Geometry: see drawing. Coordinates: mm, zero at the bounding-box minimum. Coordinates: 2 decimals unless noted, no trailing zeros. Loops run counter-clockwise (first coordinate to the right, second up) from the corner with the lowest first, then second, coordinate; pieces in that order, holes last. Notation, with made-up numbers: (64, 82.5) -> (102, 82.5) arc R4 cw to (102, 87.5) -> close; hole circle Ø10 at (-35, -36). An arc over 180 degrees is marked (long way). Put each result on its own line as item: value. Start each with the question number.
1) Cut plane B-B (z = 3.3). Return the cut outline in (x, y), plus the area to 3 significant figures.
2) Material intervals for L1, parallel to Y at x = 45, z = 3.15; L2, parallel to X at y = 4.5, z = 3.1; L3, parallel to Y at x = 18.5, z = 2.75, sorted ascending.
3) Cut plane C-C (x = 18.5). Return the cut outline in (y, z), plus the area to 3 significant figures.
4) Cut plane A-A (x = 45). Return the cut outline in (y, z).
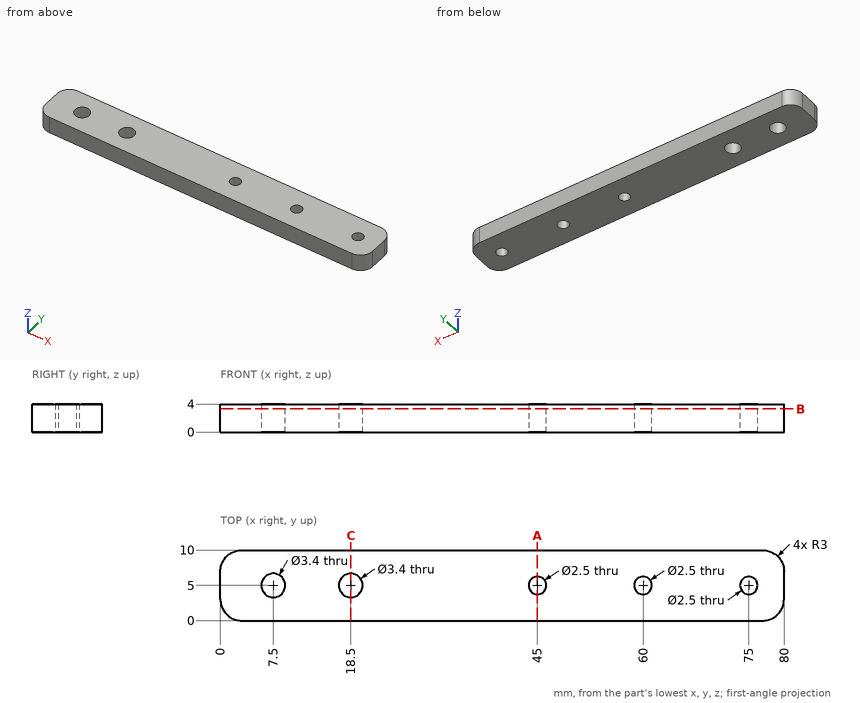
Results found:
1. outline: (0, 3) arc R3 ccw to (3, 0) -> (77, 0) arc R3 ccw to (80, 3) -> (80, 7) arc R3 ccw to (77, 10) -> (3, 10) arc R3 ccw to (0, 7) -> close; hole circle Ø3.4 at (7.5, 5); hole circle Ø3.4 at (18.5, 5); hole circle Ø2.5 at (45, 5); hole circle Ø2.5 at (60, 5); hole circle Ø2.5 at (75, 5)
1. area: 759 mm2
2. L1: y = 0 to 3.75, 6.25 to 10
2. L2: x = 0 to 5.88, 9.12 to 16.88, 20.12 to 43.85, 46.15 to 58.85, 61.15 to 73.85, 76.15 to 80
2. L3: y = 0 to 3.3, 6.7 to 10
3. outline: (0, 0) -> (3.3, 0) -> (3.3, 4) -> (0, 4) -> close; (6.7, 0) -> (10, 0) -> (10, 4) -> (6.7, 4) -> close
3. area: 26.4 mm2
4. outline: (0, 0) -> (3.75, 0) -> (3.75, 4) -> (0, 4) -> close; (6.25, 0) -> (10, 0) -> (10, 4) -> (6.25, 4) -> close
